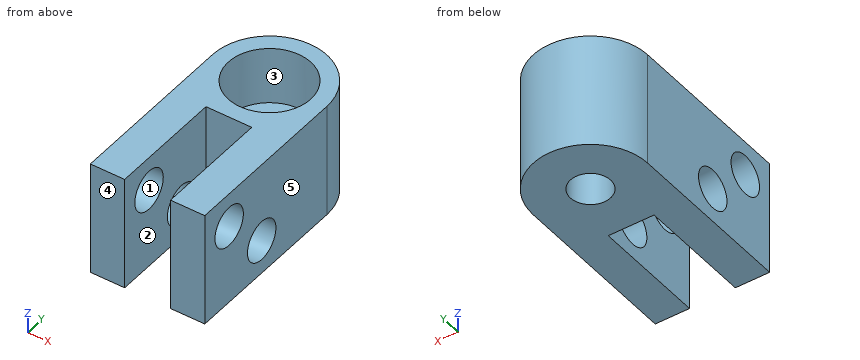
```python
from build123d import *

# Parameters (mm, degrees)
ESBO_O1_R                = 5
ESBO_O1_R_2              = 1.75
RESSALTO_EXTRUS_O1_DEPTH = 10
ESBO_O2_R                = 3.6
CORTE_EXTRUS_O1_DEPTH    = 5
RESSALTO_EXTRUS_O2_START = -10
RESSALTO_EXTRUS_O2_DEPTH = 10
ESBO_O4_R                = 1.75
CORTE_EXTRUS_O2_DEPTH    = 10


with BuildPart() as part:
    # Esboço1 → Ressalto-extrusão1 (new body)
    with BuildSketch(Plane.XY):
        Circle(ESBO_O1_R)
        Circle(ESBO_O1_R_2, mode=Mode.SUBTRACT)
    extrude(amount=RESSALTO_EXTRUS_O1_DEPTH)

    # Esboço2 → Corte-extrusão1 (cut)
    with BuildSketch(Plane.XY.offset(10)):
        Circle(ESBO_O2_R)
    extrude(amount=-CORTE_EXTRUS_O1_DEPTH, mode=Mode.SUBTRACT)

    # Esboço3 → Ressalto-extrusão2 (add)
    with BuildSketch(Plane.XY.offset(10).offset(RESSALTO_EXTRUS_O2_START)):
        with BuildLine():
            Line((2, -4.582575695), (2, -5))
            Line((2, -5), (2, -15))
            Line((2, -15), (5, -15))
            Line((5, -15), (5, 0))
            ThreePointArc((5, 0), (4.183300133, -2.738612788), (2, -4.582575695))
        make_face()
        with BuildLine():
            Line((-2, -15), (-2, -5))
            Line((-2, -5), (-2, -4.582575695))
            ThreePointArc((-2, -4.582575695), (-4.183300133, -2.738612788), (-5, 0))
            Line((-5, 0), (-5, -15))
            Line((-5, -15), (-2, -15))
        make_face()
        with BuildLine():
            Line((-2, -5), (3e-09, -5))
            ThreePointArc((3e-09, -5), (-1.021548217, -4.894531565), (-2, -4.582575695))
            Line((-2, -4.582575695), (-2, -5))
        make_face()
        with BuildLine():
            Line((3e-09, -5), (2, -5))
            Line((2, -5), (2, -4.582575695))
            ThreePointArc((2, -4.582575695), (1.02154822, -4.894531564), (3e-09, -5))
        make_face()
        with BuildLine():
            ThreePointArc((-2, -4.582575695), (-1.021548217, -4.894531565), (3e-09, -5))
            ThreePointArc((3e-09, -5), (1.02154822, -4.894531564), (2, -4.582575695))
            Line((2, -4.582575695), (-2, -4.582575695))
        make_face()
    extrude(amount=RESSALTO_EXTRUS_O2_DEPTH)

    # Esboço4 → Corte-extrusão2 (cut)
    with BuildSketch(Plane.ZY.offset(5)):
        with Locations((7, -12)):
            Circle(ESBO_O4_R)
        with Locations((3, -8)):
            Circle(ESBO_O4_R)
    extrude(amount=-CORTE_EXTRUS_O2_DEPTH, mode=Mode.SUBTRACT)


solid = part.part
```
The model under review builds one solid part; all positions refer to its coordinate system, in mm. Face numbers are marked on the shaded views. A direction names the side the tool comes from. Give positions to 0.01 mm unless a question says otherwise; leave off trailing zeros. Write each loop counter-clockwise with the first axis right and the second up, starting at its lowest first coordinate (ties: lowest second). Pieces come first, ordered by that corner, then holes.
(1) The part is to be moulded in two halves that separate along X. For the marked faces 3, 4 and 5, say which applies: released by +X, released by -X, zero draft, split by the parting line, or undercut.
(2) Consider section A-A, the plane z = 7. Give the boundary of the cut face in (x, y).
(3) For P1, Ø5.5, axis at x = 0, y = 0, coming from the +Z side; P2, Ø2, axis at x = 2, z = 2.5, coming from the +Y side, all flat-tipped, find the tip position at first contact; note any pin that passes through.
(4) Tool access review of the marked faces 1 and 2: name each direction out of +Z, -Z, +X, -X, +Y, -Y from which nothing blocks a thin tool from reaching the whole face with its end or side.
(5) Consider section C-C, the plane z = 3. Give the boundary of the cut face in (x, y), and give its area (3 significant figures).
(6) Consider section D-D, the plane y = -0.5. Give the boundary of the cut face in (x, z), and give its area (3 significant figures).
(7) To check wall thickness, follow L1, parallel to X at y = -9.75, z = 8.5; L2, parallel to Y at x = 0, z = 3.05; L3, parallel to Y at x = -2.75, z = 7. State the ranges of each line that lie inside material, in increasing order.
(8) Consider section B-B, the plane y = -12. Give the boundary of the cut face in (x, z).
Returned:
1. face 3: undercut
1. face 4: zero draft
1. face 5: released by +X
2. outline: (-5, -15) - (-2, -15) - (-2, -13.75) - (-5, -13.75) - close; (-5, -10.25) - (-2, -10.25) - (-2, -5) - (2, -5) - (2, -10.25) - (5, -10.25) - (5, 0) arc R5 ccw to (-5, 0) - close; (2, -15) - (5, -15) - (5, -13.75) - (2, -13.75) - close; hole circle Ø7.2 at (0, 0)
3. P1: stops at z = 5
3. P2: stops at y = 4.9
4. face 1: +X, -X
4. face 2: +Z, -Z, -Y
5. outline: (-5, -15) - (-2, -15) - (-2, -9.75) - (-5, -9.75) - close; (-5, -6.25) - (-2, -6.25) - (-2, -5) - (2, -5) - (2, -6.25) - (5, -6.25) - (5, 0) arc R5 ccw to (-5, 0) - close; (2, -15) - (5, -15) - (5, -9.75) - (2, -9.75) - close; hole circle Ø3.5 at (0, 0)
5. area: 119 mm2
6. outline: (-5, 0) - (-1.68, 0) - (-1.68, 5) - (-3.57, 5) - (-3.57, 10) - (-5, 10) - close; (1.68, 0) - (5, 0) - (5, 10) - (3.57, 10) - (3.57, 5) - (1.68, 5) - close
6. area: 47.6 mm2
7. L1: x = -5 to -2, 2 to 5
7. L2: y = -5 to -1.75, 1.75 to 5
7. L3: y = -15 to -13.75, -10.25 to -2.32, 2.32 to 4.18
8. outline: (-5, 0) - (-2, 0) - (-2, 5.25) - (-5, 5.25) - close; (-5, 8.75) - (-2, 8.75) - (-2, 10) - (-5, 10) - close; (2, 0) - (5, 0) - (5, 5.25) - (2, 5.25) - close; (2, 8.75) - (5, 8.75) - (5, 10) - (2, 10) - close
